```python
from build123d import *

# Parameters (mm, degrees)
BOSS_EXTRUDE1_DEPTH      = 3
BOSS_EXTRUDE2_DEPTH      = 8
CHAMFER1_SIZE            = 4
M3X0_5_TAPPED_HOLE1_D    = 2.5
CHAMFER1_OF_MIRROR1_SIZE = 4
BOSS_EXTRUDE3_REACH      = 34.14
SKETCH7_W                = 8
SKETCH7_H                = 14.15
SKETCH7_R                = 1.25
SKETCH8_R                = 5
BOSS_EXTRUDE4_DEPTH      = 12
CUT_EXTRUDE1_START       = -1
SKETCH9_R                = 5
SKETCH9_R_2              = 3
CUT_EXTRUDE1_DEPTH       = 1
SKETCH12_W               = 15.25
SKETCH12_H               = 27
BOSS_EXTRUDE5_DEPTH      = 3
M4X0_7_TAPPED_HOLE1_D    = 3.3
M5_CLEARANCE_HOLE3_D     = 5.5
DELETEFACE1_START        = 2
DELETEFACE1_DEPTH        = 8
MOVE_FACE1_BY            = 4


# Read off the part's stored shape, not the designer's step: DeleteFace1
with BuildPart() as part:
    # Sketch1 → Boss-Extrude1 (new body)
    with BuildSketch(Plane(origin=(0, 0, 0), x_dir=(1, 0, 0), z_dir=(0, 1, 0))):
        Polygon((19.75, 10), (19.75, -10), (-19.75, -10), (-19.75, 10), (-19.75, 17), (19.75, 17), align=None)
    extrude(amount=BOSS_EXTRUDE1_DEPTH)

    # Sketch4 → Boss-Extrude2 (add)
    with BuildSketch(Plane.XY.offset(10)):
        with BuildLine():
            Line((1.46, 17.15), (1.46, 3))
            Line((1.46, 3), (8.960000005, 3))
            ThreePointArc((8.960000005, 3), (4.916271098, 6.571133381), (7.96, 11.02539555))
            Line((7.96, 11.02539555), (7.96, 17.15))
            Line((7.96, 17.15), (1.46, 17.15))
        make_face()
        with BuildLine():
            ThreePointArc((13.035, 7.075), (11.841460135, 4.193539869), (8.960000005, 3))
            Line((8.960000005, 3), (16.46, 3))
            Line((16.46, 3), (16.46, 17.15))
            Line((16.46, 17.15), (9.96, 17.15))
            Line((9.96, 17.15), (9.96, 11.02539555))
            ThreePointArc((9.96, 11.02539555), (12.175635629, 9.578060627), (13.035, 7.075))
        make_face()
    boss_extrude2 = extrude(amount=-BOSS_EXTRUDE2_DEPTH)

    # Chamfer1
    # the kernel refuses this chamfer: 4 mm, written as the material it adds along each edge
    with BuildSketch(Plane(origin=(16.46, 3, 10), x_dir=(0.9996219169112968, -0.027495876610586917, 0), z_dir=(0, 0, -1))) as chamfer1_piece_1_section:
        Polygon((CHAMFER1_SIZE * 0.999621916911, -CHAMFER1_SIZE * 0.0274958766106), (-CHAMFER1_SIZE * 0.0274958766106, -CHAMFER1_SIZE * 0.999621916911), (0, 0), align=None)
    chamfer1_piece_1 = extrude(amount=8, mode=Mode.PRIVATE)
    chamfer1_piece_1 = split(chamfer1_piece_1, bisect_by=Plane(origin=(19.75, 4.372732245, 6), z_dir=(-1, 0, 0)), keep=Keep.TOP, mode=Mode.PRIVATE)
    add(chamfer1_piece_1)

    # M3x0.5 Tapped Hole1 (through all)
    with Locations(Plane.ZY.offset(-1.46)):
        with Locations((6, 14.087697775)):
            m3x0_5_tapped_hole1 = Hole(M3X0_5_TAPPED_HOLE1_D / 2)

    # Mirror1: Boss-Extrude2, M3x0.5 Tapped Hole1 across plane
    add(boss_extrude2.mirror(Plane(origin=(0, 0, 0), x_dir=(0, 0, 1), z_dir=(1, 0, 0))))
    add(m3x0_5_tapped_hole1.mirror(Plane(origin=(0, 0, 0), x_dir=(0, 0, 1), z_dir=(1, 0, 0))), mode=Mode.SUBTRACT)

    # Chamfer1 of Mirror1
    # the kernel refuses this chamfer: 4 mm, written as the material it adds along each edge
    with BuildSketch(Plane(origin=(-16.46, 3, 10), x_dir=(-0.9996219169112968, -0.027495876610586917, 0), z_dir=(0, 0, -1))) as chamfer1_of_mirror1_piece_1_section:
        Polygon((CHAMFER1_OF_MIRROR1_SIZE * 0.999621916911, CHAMFER1_OF_MIRROR1_SIZE * 0.0274958766106), (-CHAMFER1_OF_MIRROR1_SIZE * 0.0274958766106, CHAMFER1_OF_MIRROR1_SIZE * 0.999621916911), (0, 0), align=None)
    chamfer1_of_mirror1_piece_1 = extrude(amount=8, mode=Mode.PRIVATE)
    chamfer1_of_mirror1_piece_1 = split(chamfer1_of_mirror1_piece_1, bisect_by=Plane(origin=(-19.75, 4.372732245, 6), z_dir=(1, 0, 0)), keep=Keep.TOP, mode=Mode.PRIVATE)
    add(chamfer1_of_mirror1_piece_1)

    # Sketch7 → Boss-Extrude3 (add, up to next)
    with BuildSketch(Plane(origin=(-1.46, 0, 0), x_dir=(0, 0, -1), z_dir=(1, 0, 0)), mode=Mode.PRIVATE) as boss_extrude3_sk1:
        with Locations((-6, 10.075)):
            Rectangle(SKETCH7_W, SKETCH7_H)
        with Locations(Location((-6, 14.087697775, 0), (0, 0, 180))):
            Circle(SKETCH7_R, mode=Mode.SUBTRACT)
    boss_extrude3_tool1 = extrude(boss_extrude3_sk1.sketch, amount=BOSS_EXTRUDE3_REACH, mode=Mode.PRIVATE) - part.part
    add(boss_extrude3_tool1.solids().sort_by_distance((-1.46, 9.893108, 6))[0])

    # Sketch8 → Boss-Extrude4 (add)
    with BuildSketch(Plane(origin=(0, 3, 0), x_dir=(1, 0, 0), z_dir=(0, 1, 0))):
        with Locations(Location((-5.96, 5, 0), (0, 0, 90))):
            Circle(SKETCH8_R)
        with Locations(Location((5.96, 5, 0), (0, 0, 90))):
            Circle(SKETCH8_R)
        with Locations(Location((-19.554616806, 11.339273926, 0), (0, 0, 92.239496679))):
            Circle(SKETCH8_R)
        with Locations(Location((19.554616806, 11.339273926, 0), (0, 0, 87.760503321))):
            Circle(SKETCH8_R)
    extrude(amount=BOSS_EXTRUDE4_DEPTH)

    # Sketch9 → Cut-Extrude1 (cut)
    # profile 1 of 4: a face of its own
    with BuildSketch(Plane(origin=(0, 15, 0), x_dir=(1, 0, 0), z_dir=(0, 1, 0)).offset(CUT_EXTRUDE1_START)):
        with Locations(Location((5.96, 5, 0), (0, 0, 90))):
            Circle(SKETCH9_R)
        with Locations(Location((5.96, 5, 0), (0, 0, 270))):
            Circle(SKETCH9_R_2, mode=Mode.SUBTRACT)
    # profile 2 of 4: a face of its own
    with BuildSketch(Plane(origin=(0, 15, 0), x_dir=(1, 0, 0), z_dir=(0, 1, 0)).offset(CUT_EXTRUDE1_START)):
        with Locations(Location((-5.96, 5, 0), (0, 0, 90))):
            Circle(SKETCH9_R)
        with Locations(Location((-5.96, 5, 0), (0, 0, 270))):
            Circle(SKETCH9_R_2, mode=Mode.SUBTRACT)
    # profile 3 of 4: a face of its own
    with BuildSketch(Plane(origin=(0, 15, 0), x_dir=(1, 0, 0), z_dir=(0, 1, 0)).offset(CUT_EXTRUDE1_START)):
        with Locations(Location((-19.554616806, 11.339273926, 0), (0, 0, 92.239496679))):
            Circle(SKETCH9_R)
        with Locations(Location((-19.554616806, 11.339273926, 0), (0, 0, 270))):
            Circle(SKETCH9_R_2, mode=Mode.SUBTRACT)
    # profile 4 of 4: a face of its own
    with BuildSketch(Plane(origin=(0, 15, 0), x_dir=(1, 0, 0), z_dir=(0, 1, 0)).offset(CUT_EXTRUDE1_START)):
        with Locations(Location((19.554616806, 11.339273926, 0), (0, 0, 87.760503321))):
            Circle(SKETCH9_R)
        with Locations(Location((19.554616806, 11.339273926, 0), (0, 0, 270))):
            Circle(SKETCH9_R_2, mode=Mode.SUBTRACT)
    extrude(amount=CUT_EXTRUDE1_DEPTH, mode=Mode.SUBTRACT)

    # Sketch12 → Boss-Extrude5 (add)
    with BuildSketch(Plane.XZ):
        with Locations((-27.375, -3.5)):
            Rectangle(SKETCH12_W, SKETCH12_H)
        with Locations((27.375, -3.5)):
            Rectangle(SKETCH12_W, SKETCH12_H)
    extrude(amount=-BOSS_EXTRUDE5_DEPTH)

    # M4x0.7 Tapped Hole1 (through all)
    with Locations(Plane.XZ):
        with Locations((-5.96, -5), (5.96, -5), (-19.554616806, -11.339273926), (19.554616806, -11.339273926)):
            Hole(M4X0_7_TAPPED_HOLE1_D / 2)

    # M5 Clearance Hole3 (through all)
    with Locations(Plane(origin=(0, 3, 0), x_dir=(1, 0, 0), z_dir=(0, 1, 0))):
        with Locations((25, 0), (-25, 0)):
            Hole(M5_CLEARANCE_HOLE3_D / 2)

    # DeleteFace1 outline → DeleteFace1 (add)
    with BuildSketch(Plane.XY.offset(DELETEFACE1_START)):
        Polygon((-20.46, 3), (-19.75, 3), (-19.75, 3.71), align=None)
        Polygon((20.46, 3), (19.75, 3.71), (19.75, 3), align=None)
    extrude(amount=DELETEFACE1_DEPTH)

    # Move Face1: a face moved outward by 4.0
    extrude(part.faces().sort_by_distance((0, 0, -3.503622632))[0], amount=MOVE_FACE1_BY, dir=(0, -1, 0))


solid = part.part
```
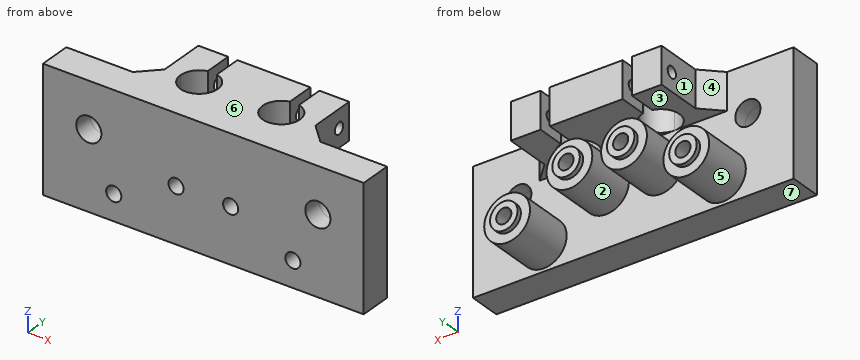
Check sheet for the modelled part. Datum: model origin and axes. Units: mm. Face numbers are marked on the shaded views. A direction names the side the tool comes from. Coordinates: 2 decimals unless noted, no trailing zeros. Order: outer loops, then holes, each group sorted by start corner. A loop starts at its lowest first (then second) coordinate and runs counter-clockwise, first axis right, second up. Notation, with made-up numbers: (55.5, 24) -> (80.5, 24) arc R27 cw to (80.5, 51) -> close; hole circle Ø11 at (-13.75, 21.25). An arc over 180 degrees is marked (long way). Write item = value, one per line. Start each with the question number.
1) Cross-section at A-A (z = 6). State how many separate pieces and enclosed holes the cut face has, then the cut area to 3 significant figures.
2) Material ranges on L1, parallel to Z at x = 25, y = -1.95; L2, parallel to X at y = -1, z = -0.5; L3, parallel to X at y = 2.5, z = -11.25, recorded low to high.
3) Access from +Z, -Z, +X, -X, +Y, -Y to the whole of each face (thin tool, end or side, straight path). Record for the marked faces 1, 2 and 3.
4) Mould release check, pull along Z, two halves, no side actions. Record for the marked faces 4, 5, 6 and 7: +Z half, -Z half, draft (parallel to the pull), parting line (faces both ways), or undercut.
5) Go/stop test with flat-tipped pins: P1, Ø5, axis at y = 13, z = 4.5, coming from the -X side; P2, Ø3, axis at y = 11, z = -6.5, coming from the -X side; P3, Ø2, axis at y = 14.09, z = 6, coming from the -X side; P4, Ø12, axis at x = 16, y = 14, coming from the -Z side. Record where each tip stops, or that it passes through.
6) Cross-section at B-B (z = -5). Enter the section's corners in (x, y), then the cut area to 3 significant figures.
7) Cross-section at C-C (x = -5.96). Enter the section's corners in (y, z), then the cut area to 3 significant figures.
8) Cross-section at D-D (y = 2). Enter the section's corners in (x, z), then the cut area to 3 significant figures.
Ans:
q1.separate_pieces = 4
q1.enclosed_holes = 0
q1.area = 771 mm²
q2.L1 = -17 to -2.75, 2.75 to 10
q2.L2 = -35 to -27.7, -22.3 to 22.3, 27.7 to 35
q2.L3 = -35 to -21.2, -17.91 to 17.91, 21.2 to 35
q3.face_1 = +Z, -X, +Y
q3.face_2 = +Y
q3.face_3 = +X, -X, +Y
q4.face_4 = draft
q4.face_5 = undercut
q4.face_6 = +Z half
q4.face_7 = -Z half
q5.P1 = -16.46
q5.P2 = -23.28
q5.P3 = through
q5.P4 = -16.34
q6.outline = (-35, -4) -> (-7.61, -4) -> (-7.61, 15) -> (-8.96, 15) -> (-8.96, 14) -> (-10.96, 14) -> (-10.96, 3) -> (-35, 3) -> close; (-4.31, -4) -> (4.31, -4) -> (4.31, 15) -> (2.96, 15) -> (2.96, 14) -> (0.96, 14) -> (0.96, 3) -> (-0.96, 3) -> (-0.96, 14) -> (-2.96, 14) -> (-2.96, 15) -> (-4.31, 15) -> close; (7.61, -4) -> (35, -4) -> (35, 3) -> (10.96, 3) -> (10.96, 14) -> (8.96, 14) -> (8.96, 15) -> (7.61, 15) -> close
q6.area = 597 mm²
q7.outline = (-4, -17) -> (3, -17) -> (3, -10) -> (14, -10) -> (14, -8) -> (15, -8) -> (15, -6.65) -> (-4, -6.65) -> close; (-4, -3.35) -> (15, -3.35) -> (15, -2) -> (14, -2) -> (14, 0) -> (3, 0) -> (3, 2) -> (4.32, 2) -> (4.32, 10) -> (-4, 10) -> close; (9.83, 2) -> (17.15, 2) -> (17.15, 10) -> (9.83, 10) -> close; hole circle Ø2.5 at (14.09, 6)
q7.area = 306 mm²
q8.outline = (-35, -17) -> (35, -17) -> (35, 10) -> (-35, 10) -> close; hole circle Ø5.5 at (-25, 0); hole circle Ø3.3 at (-19.55, -11.34); hole circle Ø3.3 at (-5.96, -5); hole circle Ø3.3 at (5.96, -5); hole circle Ø3.3 at (19.55, -11.34); hole circle Ø5.5 at (25, 0)
q8.area = 1,810 mm²
